CAD build for the part. Positions are in the model's coordinates, mm. Round coordinates to 2 decimals unless told otherwise and drop trailing zeros. Order: outer loops, then holes, each group sorted by start corner. A loop starts at its lowest first (then second) coordinate and runs counter-clockwise, first axis right, second up. Notation, with made-up numbers: M 25,4.25 L 83,4.25 A26 ccw 83,30.25 Z; hole C 16,39.5 d3. An arc over 180 degrees is marked long. Put each result on its own line as item: value.
```python
from build123d import *

# Parameters (mm, degrees)
SKETCH021_R   = 8.5
SKETCH021_R_2 = 4.5
PAD023_DEPTH  = 1


with BuildPart() as clone_of_spacer:
    # Sketch021 → Pad023 (new body)
    with BuildSketch(Plane.XY.offset(29)):
        with Locations((-23, 23)):
            Circle(SKETCH021_R)
        with Locations((-23, 23)):
            Circle(SKETCH021_R_2, mode=Mode.SUBTRACT)
    extrude(amount=PAD023_DEPTH)


with BuildPart() as part_mirroring042:
    # Part__Mirroring042: instance of Clone of spacer
    add(clone_of_spacer.part.mirror(Plane(origin=(0, 0, 0), x_dir=(1, 0, 0), z_dir=(0, 1, 0))))


with BuildPart() as part_mirroring044:
    # Part__Mirroring044: instance of Part__Mirroring042
    add(part_mirroring042.part.mirror(Plane(origin=(0, 0, 0), x_dir=(0, -1, 0), z_dir=(1, 0, 0))))


solid = part_mirroring044.part
```
Item 1: Probe line 1 along Y through (x, z) = (23, 29.55); line 2 along X through (y, z) = (-23, 29.4); line 3 along X through (y, z) = (-25.75, 29.8). List the from-to ranges inside material, lowest first. Write a range as [from, to].
Answers below:
line 1: [-31.5, -27.5], [-18.5, -14.5]
line 2: [14.5, 18.5], [27.5, 31.5]
line 3: [14.96, 19.44], [26.56, 31.04]
Item 2: Band-saw the part on D-D on y = -29.25. Give the cut face in (x, z), and give its area (3 significant figures).
Answers below:
outline: M 17.24,29 L 28.76,29 L 28.76,30 L 17.24,30 Z
area: 11.5 mm²
Item 3: Band-saw the part on B-B on y = -23. Give the cut face in (x, z), and give its area (3 significant figures).
Answers below:
outline: M 14.5,29 L 18.5,29 L 18.5,30 L 14.5,30 Z; M 27.5,29 L 31.5,29 L 31.5,30 L 27.5,30 Z
area: 8.00 mm²
Item 4: Mould opens along Y. For faces 1 (the cylindrical face through (24.84, -14.7, 29.49)), 2 (the flat face through (19, -19, 29)), 3 (the cylindrical face through (26.32, -26.04, 29.49)) say: pulls with the +Y half, pulls with the -Y half, needs draft (parallel to the pull), parting line crosses it, or undercut.
Answers below:
face 1: parting line crosses it
face 2: needs draft
face 3: undercut
Item 5: Band-saw the part on C-C on z = 29.2. Give the cut face in (x, y).
Answers below:
outline: C 23,-23 d17; hole C 23,-23 d9
Item 6: Pin check, flat tip, straight feed: P1, Ø2, axis at x = 22, y = -21.5, coming from the -Z side. Stop position of the tip, or through.
Answers below:
P1: through
Item 7: Band-saw the part on A-A on x = 23. Give the cut face in (y, z).
Answers below:
outline: M -31.5,29 L -27.5,29 L -27.5,30 L -31.5,30 Z; M -18.5,29 L -14.5,29 L -14.5,30 L -18.5,30 Z
